Verification items for the finished model (mm, model axes). A direction names the side the tool comes from. Round coordinates to 2 decimals unless told otherwise and drop trailing zeros. Order: outer loops, then holes, each group sorted by start corner. A loop starts at its lowest first (then second) coordinate and runs counter-clockwise, first axis right, second up. Notation, with made-up numbers: M 63.25,-15 L 69.25,-15 A18 cw 69.25,15 Z; hole C 71,25.25 d2. An arc over 180 degrees is marked long. Use one line per item in the form item = value. Start each with the question number.
Item 1: Go/stop test with a flat-tipped pin: pin 1 Ø3 at (y, z) = (-4, 32.5) entering from +X. Record where the tip stops, or that it passes through.
Item 2: Thickness scan on probe 1 along Y at (x, z) = (3.5, -10); probe 2 along X at (y, z) = (-1, -6); probe 3 along Y at (x, z) = (6.5, 25). Record the ranges inside material, lowest first. Write a range as [from, to].
Item 3: Cross-section at B-B on z = 30. Enter the section's corners in (x, y).
Item 4: Cross-section at C-C on z = -31. Enter the section's corners in (x, y), then the cut area to 3 significant figures.
Item 5: Cross-section at A-A on y = -2. Enter the section's corners in (x, z).
Item 6: Tool access check on faces 1 (the flat face through (0, -2, 30)), 2 (the flat face through (-19, -8, -40)). Record the directions out of +Z, -Z, +X, -X, +Y, -Y that give a thin tool (end or side, any length) a straight path to the whole face; none if there is none.
Item 7: Release check for a two-part mould opening along Z. For faces 3 (the flat face through (0, -2, -30)), 4 (the flat face through (-19, -8, 40)), 5 (the flat face through (-50, -7, -1)) record: +Z half, -Z half, draft (parallel to the pull), parting line (faces both ways), or undercut.
from build123d import *

# Parameters (mm, degrees)
BOSS_EXTRUDE1_DEPTH = 12
SKETCH2_W           = 80
SKETCH2_H           = 15
BOSS_EXTRUDE2_DEPTH = 50


with BuildPart() as part:
    # Sketch1 → Boss-Extrude1 (new body)
    with BuildSketch(Plane(origin=(0, 0, 0), x_dir=(0, 0, -1), z_dir=(1, 0, 0))):
        with BuildLine():
            Line((40, 0), (36.5, 0))
            ThreePointArc((36.5, 0), (30, -6.5), (23.5, 0))
            Line((23.5, 0), (16.5, 0))
            ThreePointArc((16.5, 0), (10, -6.5), (3.5, 0))
            Line((3.5, 0), (-3.5, 0))
            ThreePointArc((-3.5, 0), (-10, -6.5), (-16.5, 0))
            Line((-16.5, 0), (-23.5, 0))
            ThreePointArc((-23.5, 0), (-30, -6.5), (-36.5, 0))
            Line((-36.5, 0), (-40, 0))
            Line((-40, 0), (-40, -15))
            Line((-40, -15), (40, -15))
            Line((40, -15), (40, 0))
        make_face()
    extrude(amount=BOSS_EXTRUDE1_DEPTH)

    # Sketch2 → Boss-Extrude2 (add)
    with BuildSketch(Plane.ZY):
        with Locations((0, -7.5)):
            Rectangle(SKETCH2_W, SKETCH2_H)
    extrude(amount=BOSS_EXTRUDE2_DEPTH)


solid = part.part
Output values:
q1.pin_1 = 0
q2.probe_1 = [-15, -6.5]
q2.probe_2 = [-50, 0]
q2.probe_3 = [-15, -4.15]
q3.outline = M -50,-15 L 12,-15 L 12,-6.5 L 0,-6.5 L 0,0 L -50,0 Z
q4.outline = M -50,-15 L 12,-15 L 12,-6.42 L 0,-6.42 L 0,0 L -50,0 Z
q4.area = 853 mm2
q5.outline = M -50,-40 L 12,-40 L 12,-36.18 L 0,-36.18 L 0,-23.82 L 12,-23.82 L 12,-16.18 L 0,-16.18 L 0,-3.82 L 12,-3.82 L 12,3.82 L 0,3.82 L 0,16.18 L 12,16.18 L 12,23.82 L 0,23.82 L 0,36.18 L 12,36.18 L 12,40 L -50,40 Z
q6.face_1 = +X, +Y
q6.face_2 = -Z, +X, -X, +Y, -Y
q7.face_3 = undercut
q7.face_4 = +Z half
q7.face_5 = draft
